Design review of the part built by this model. Coordinates are the model's own, in mm. A direction names the side the tool comes from. Give positions to 0.01 mm unless a question says otherwise; leave off trailing zeros. Loops run counter-clockwise (first coordinate to the right, second up) from the corner with the lowest first, then second, coordinate; pieces in that order, holes last.
from build123d import *

# Parameters (mm, degrees)
SKETCH1_W           = 20
SKETCH1_H           = 20
SKETCH1_W_2         = 17
SKETCH1_H_2         = 17
BOSS_EXTRUDE1_DEPTH = 160
SKETCH2_R           = 2.125
CUT_EXTRUDE1_DEPTH  = 162.554944214
SKETCH3_R           = 2.125
CUT_EXTRUDE2_DEPTH  = 162.554944214


with BuildPart() as part:
    # Sketch1 → Boss-Extrude1 (new body)
    with BuildSketch(Plane.XY):
        Rectangle(SKETCH1_W, SKETCH1_H)
        Rectangle(SKETCH1_W_2, SKETCH1_H_2, mode=Mode.SUBTRACT)
    extrude(amount=-BOSS_EXTRUDE1_DEPTH)

    # Sketch2 → Cut-Extrude1 (cut, through all)
    with BuildSketch(Plane(origin=(0, 10, 0), x_dir=(1, 0, 0), z_dir=(0, 1, 0))):
        with Locations(Location((0, 33.375, 0), (0, 0, 270))):
            Circle(SKETCH2_R)
        with Locations(Location((0, 129.8, 0), (0, 0, 270))):
            Circle(SKETCH2_R)
    extrude(amount=-CUT_EXTRUDE1_DEPTH, mode=Mode.SUBTRACT)

    # Sketch3 → Cut-Extrude2 (cut, through all)
    with BuildSketch(Plane.ZY.offset(10)):
        with Locations((-43.375, 0)):
            Circle(SKETCH3_R)
        with Locations((-119.8, 0)):
            Circle(SKETCH3_R)
    extrude(amount=-CUT_EXTRUDE2_DEPTH, mode=Mode.SUBTRACT)


solid = part.part
Q1. Draft analysis for pull direction X (two halves, no side actions). For faces 1 (the face through (10, 0, -79)), 2 (the face through (0.64, 9.26, -31.35)), 3 (the face through (-8.5, 0, -79)), 4 (the face through (-9, 0, 0)), state which applies: pulls with the +X half, pulls with the -X half, needs draft (parallel to the pull), parting line crosses it, or undercut.
Results:
face 1: pulls with the +X half
face 2: undercut
face 3: undercut
face 4: needs draft
Q2. Take a section at B-B (x = 5). Give the boundary of the cut face in (y, z).
Results:
outline: (-10, -160) - (-8.5, -160) - (-8.5, 0) - (-10, 0) - close; (8.5, -160) - (10, -160) - (10, 0) - (8.5, 0) - close
Q3. Take a section at C-C (y = 0). Give the boundary of the cut face in (x, z) (3 decimals).
Results:
outline: (-10, -160) - (-8.5, -160) - (-8.5, -121.925) - (-10, -121.925) - close; (-10, -117.675) - (-8.5, -117.675) - (-8.5, -45.5) - (-10, -45.5) - close; (-10, -41.25) - (-8.5, -41.25) - (-8.5, 0) - (-10, 0) - close; (8.5, -160) - (10, -160) - (10, -121.925) - (8.5, -121.925) - close; (8.5, -117.675) - (10, -117.675) - (10, -45.5) - (8.5, -45.5) - close; (8.5, -41.25) - (10, -41.25) - (10, 0) - (8.5, 0) - close
Q4. Wall thickness on line 1 (X direction, y = -5.25, z = -56); line 2 (X direction, y = -9.35, z = -129.8) (3 decimals): over which ranges is each line inside the solid? List them lowest first.
Results:
line 1: x = -10 to -8.5, 8.5 to 10
line 2: x = -10 to -2.125, 2.125 to 10
Q5. Take a section at D-D (z = -148). Give the boundary of the cut face in (x, y).
Results:
outline: (-10, -10) - (10, -10) - (10, 10) - (-10, 10) - close; hole (-8.5, -8.5) - (8.5, -8.5) - (8.5, 8.5) - (-8.5, 8.5) - close
Q6. Tool access review of faces 5 (the face through (0, -8.5, -79)), 6 (the face through (0.64, -9.24, -31.35)): name each direction out of +Z, -Z, +X, -X, +Y, -Y from which nothing blocks a thin tool from reaching the whole face with its end or side.
Results:
face 5: +Z, -Z
face 6: +Y, -Y
Q7. Take a section at A-A (z = -129.8). Give the boundary of the cut face in (x, y) (3 decimals).
Results:
outline: (-10, -10) - (-2.125, -10) - (-2.125, -8.5) - (-8.5, -8.5) - (-8.5, 8.5) - (-2.125, 8.5) - (-2.125, 10) - (-10, 10) - close; (2.125, -10) - (10, -10) - (10, 10) - (2.125, 10) - (2.125, 8.5) - (8.5, 8.5) - (8.5, -8.5) - (2.125, -8.5) - close
Q8. Insertion check: pin 1 (3.5 mm diameter, centred on y = 0, z = -119.8, fed in from +X). The pin has a flat end and moves straight along its axis. Give the tip position at first contact, or say it passes through.
Results:
pin 1: passes through
